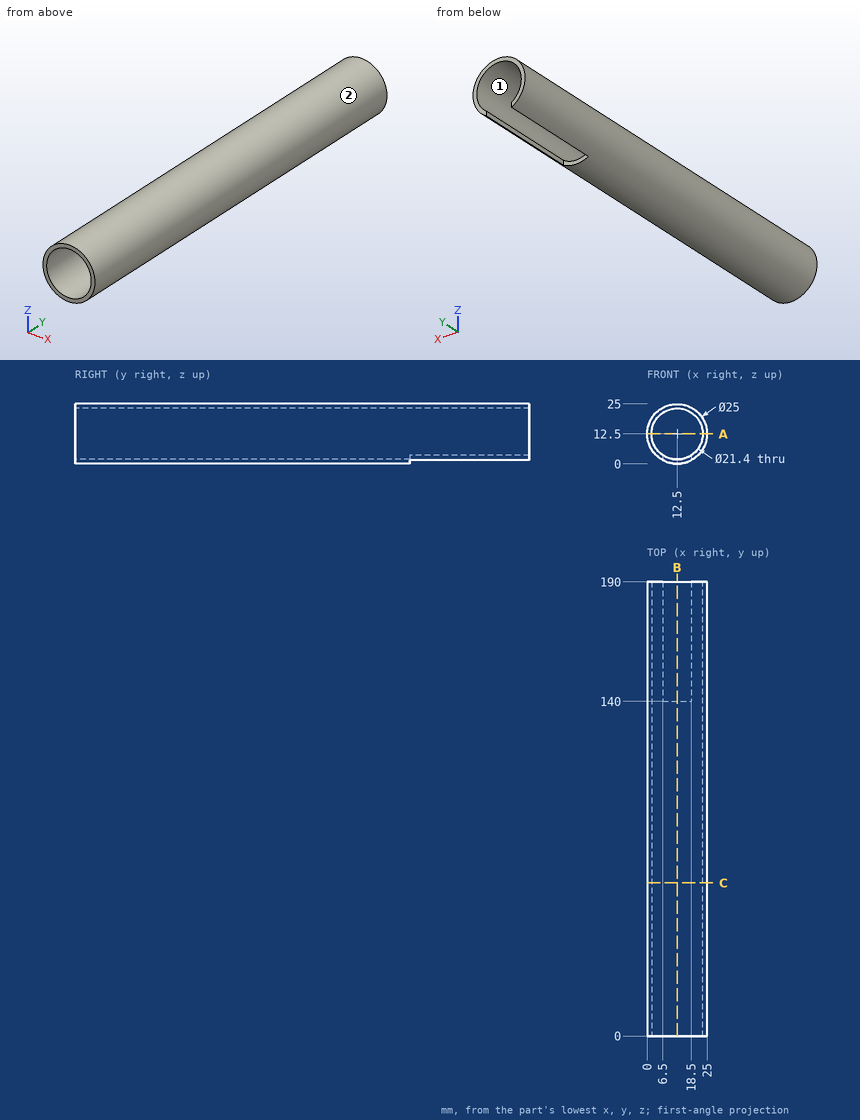
Study the drawing (mm; zero at the part's minimum x, y, z) and answer. Coordinates: 2 decimals unless noted, no trailing zeros. Write each loop counter-clockwise with the first axis right and the second up, starting at its lowest first coordinate (ties: lowest second). Pieces come first, ordered by that corner, then holes.
Q1. Section C-C, the plane y = 64 is taken. Write down the section's boundary in (x, z).
Returned:
outline: circle Ø25 at (12.5, 12.5); hole circle Ø21.4 at (12.5, 12.5)
Q2. Section B-B, the plane x = 12.5 is taken. Write down the section's boundary in (y, z), then the cut area to 3 significant figures.
Returned:
outline: (0, 0) - (140, 0) - (140, 1.8) - (0, 1.8) - close; (0, 23.2) - (190, 23.2) - (190, 25) - (0, 25) - close
area: 594 mm2
Q3. The mould has two halves that part along X. Classify the marked faces 1 and 2: released by +X, released by -X, zero draft, split by the parting line, or undercut.
Returned:
face 1: undercut
face 2: split by the parting line
Q4. Given P1, Ø1.5, axis at y = 32, z = 21.5, coming from the +X side; P2, Ø1, axis at x = 22, y = 55, coming from the +Z side; P3, Ø3, axis at x = 15, z = 2, coming from the +Y side, each flat-ended and moving along its own axis, determine where each tip first touches the part or whether it passes through.
Returned:
P1: stops at x = 21.89
P2: stops at z = 21.17
P3: stops at y = 140
Q5. Section A-A, the plane z = 12.5 is taken. Write down the section's boundary in (x, y), then the cut area to 3 significant figures.
Returned:
outline: (0, 0) - (1.8, 0) - (1.8, 190) - (0, 190) - close; (23.2, 0) - (25, 0) - (25, 190) - (23.2, 190) - close
area: 684 mm2
Q6. Find the intervals of material crossed by line 1 along X through (y, z) = (149, 12.5); line 2 along X through (y, z) = (71.5, 9), in increasing order.
Returned:
line 1: x = 0 to 1.8, 23.2 to 25
line 2: x = 0.5 to 2.39, 22.61 to 24.5
